Input: dimensioned drawing with shaded views. Units: mm. Origin: part minimum x, y, z. A direction names the side the tool comes from. Give positions to 0.01 mm unless a question says otherwise; leave off trailing zeros. Write each loop counter-clockwise with the first axis right and the second up, starting at its lowest first coordinate (ties: lowest second). Pieces come first, ordered by that corner, then holes. Notation, with made-up numbers: (-3.75, 57) - (40.25, 57) arc R14 cw to (40.25, 68) - close; hole circle Ø10 at (42, 60.5). An arc over 180 degrees is marked (long way). Answer as CSV lines item,"result".
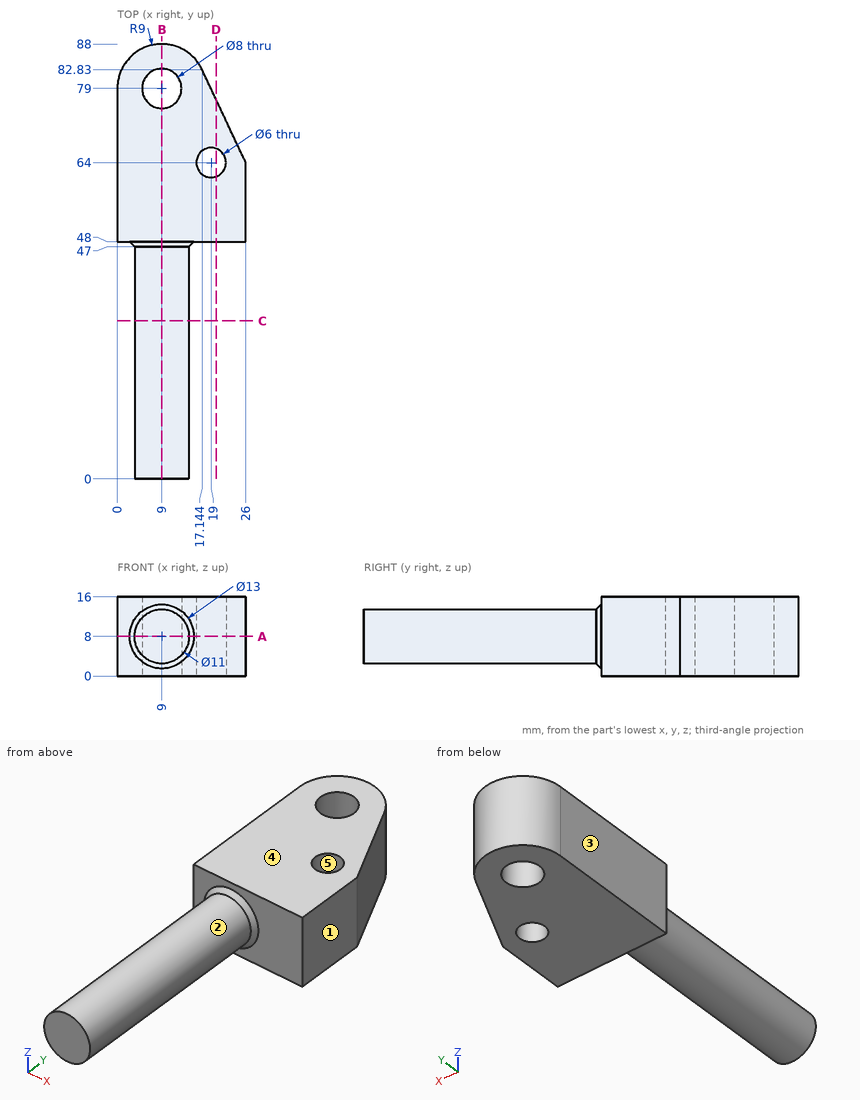
Item 1: Cut plane A-A on z = 8. Return the cut outline in (x, y), plus the area to 3 significant figures.
The answers:
outline,"(0, 48) - (2.5, 48) - (3.5, 47) - (3.5, 0) - (14.5, 0) - (14.5, 47) - (15.5, 48) - (26, 48) - (26, 64) - (17.14, 82.83) arc R9 ccw to (0, 79) - close; hole circle Ø8 at (9, 79); hole circle Ø6 at (19, 64)"
area,"1,330 mm²"
Item 2: Cut plane B-B on x = 9. Return the cut outline in (y, z).
The answers:
outline,"(0, 2.5) - (47, 2.5) - (48, 1.5) - (48, 0) - (75, 0) - (75, 16) - (48, 16) - (48, 14.5) - (47, 13.5) - (0, 13.5) - close; (83, 0) - (88, 0) - (88, 16) - (83, 16) - close"
Item 3: Cut plane D-D on x = 20. Return the cut outline in (y, z).
The answers:
outline,"(48, 0) - (61.17, 0) - (61.17, 16) - (48, 16) - close; (66.83, 0) - (76.76, 0) - (76.76, 16) - (66.83, 16) - close"
Item 4: Cut plane C-C on y = 32. Return the cut outline in (x, z).
The answers:
outline,"circle Ø11 at (9, 8)"
Item 5: Ray query, line 1 (Y direction, x = 9, z = 3.5); line 2 (Y direction, x = 21, z = 10.5) (1 decimal); line 3 (X direction, y = 82.5, z = 11) (1 decimal). Return the intervals inside material, ascending. Write a range as from..to.
The answers:
line 1,"0..75, 83..88"
line 2,"48..61.8, 66.2..74.6"
line 3,"0.7..7.1, 10.9..17.3"
Item 6: Mould query, pull axis X, two halves, no side actions, for the marked faces 3, 4 and 5. Classes: +X half, -X half, draft (parallel to the pull), parting line (faces both ways), or undercut.
The answers:
face 3,"-X half"
face 4,"draft"
face 5,"undercut"
Item 7: Contact query for flat-ended pins moving along their axis: pin 1 (8 mm diameter, centred on y = 44.5, z = 14.5, fed in from +X); pin 2 (8 mm diameter, centred on y = 41.5, z = 11, fed in from -X); pin 3 (10 mm diameter, centred on x = 12.5, y = 39.5, fed in from +Z); pin 4 (1 mm diameter, centred on x = 7.5, y = 28.5, fed in from +Z). Output: stop coordinate, or through.
The answers:
pin 1,"x = 26"
pin 2,"x = 3.5"
pin 3,"z = 13.5"
pin 4,"z = 13.41"
Item 8: Reachability of the marked faces 1 and 2 from +Z, -Z, +X, -X, +Y, -Y: full face, straight path, thin tool, end or side. Return the list, or none.
The answers:
face 1,"+Z, -Z, +X, +Y, -Y"
face 2,"-Y"
